from build123d import *

# Parameters (mm, degrees)
F1_DEPTH  = 1875
F2_W      = 2
F2_H      = 28
F3_DEPTH  = 650
F4_W      = 500
F4_H      = 400
F5_DEPTH  = 300
F6_W      = 496
F6_H      = 396
F7_DEPTH  = 300
F8_R      = 50
F9_R      = 50
F10_R     = 25
F11_DEPTH = 2
F12_R     = 12.5
F13_DEPTH = 2
F14_W     = 30
F14_H     = 30
F15_DEPTH = 920
F16_W     = 570
F16_H     = 30
F17_DEPTH = 1815


with BuildPart() as f1:
    # F0 (on Right) → F1 (new body)
    with BuildSketch(Plane.YZ):
        Polygon((0, 30), (0, 0), (700, 0), (700, 80), (680, 80), (680, 2), (30, 2), (30, 30), align=None)
    extrude(amount=F1_DEPTH)

    # F2 (on face) → F3 (join, through all)
    with BuildSketch(Plane(origin=(0, 30, 0), x_dir=(-1, 0, 0), z_dir=(0, 1, 0))):
        with Locations((-1874, 16)):
            Rectangle(F2_W, F2_H)
        with Locations((-1, 16)):
            Rectangle(F2_W, F2_H)
    extrude(amount=F3_DEPTH)

    # F4 (on face) → F5 (join)
    with BuildSketch(Plane(origin=(0, 0, 0), x_dir=(1, 0, 0), z_dir=(0, 0, -1))):
        with Locations((650, -300)):
            Rectangle(F4_W, F4_H)
        with Locations((1200, -300)):
            Rectangle(F4_W, F4_H)
    extrude(amount=F5_DEPTH)

    # F6 (on face) → F7 (cut)
    with BuildSketch(Plane.XY.offset(2)):
        with Locations((650, 300)):
            Rectangle(F6_W, F6_H)
        with Locations((1200, 300)):
            Rectangle(F6_W, F6_H)
    extrude(amount=-F7_DEPTH, mode=Mode.SUBTRACT)

    # F8
    f8_edges = [f1.edges().sort_by_distance(p)[0] for p in [
        (402, 102, -148),
        (402, 498, -148),
        (952, 498, -148),
        (1448, 498, -148),
        (898, 498, -148),
        (898, 102, -148),
        (1448, 102, -148),
        (1448, 300, -298),
        (1200, 498, -298),
        (952, 300, -298),
        (952, 102, -148),
        (1200, 102, -298),
        (650, 102, -298),
        (402, 300, -298),
        (650, 498, -298),
        (898, 300, -298),
    ]]
    fillet(f8_edges, radius=F8_R)

    # F9
    f9_edges = [f1.edges().sort_by_distance(p)[0] for p in [
        (400, 100, -150),
        (900, 100, -150),
        (950, 100, -150),
        (1450, 100, -150),
        (1450, 500, -150),
        (950, 500, -150),
        (900, 500, -150),
        (400, 500, -150),
        (400, 300, -300),
        (650, 500, -300),
        (900, 300, -300),
        (650, 100, -300),
        (950, 300, -300),
        (1200, 500, -300),
        (1450, 300, -300),
        (1200, 100, -300),
    ]]
    fillet(f9_edges, radius=F9_R)

    # F10 (on face) → F11 (cut, through all)
    with BuildSketch(Plane.XY.offset(-298)):
        with Locations((650, 373)):
            Circle(F10_R)
        with Locations((1200, 373)):
            Circle(F10_R)
    extrude(amount=-F11_DEPTH, mode=Mode.SUBTRACT)

    # F12 (on face) → F13 (cut, through all)
    with BuildSketch(Plane.XY.offset(2)):
        with Locations((560, 588)):
            Circle(F12_R)
        with Locations((740, 588)):
            Circle(F12_R)
        with Locations((1110, 588)):
            Circle(F12_R)
        with Locations((1290, 588)):
            Circle(F12_R)
    extrude(amount=-F13_DEPTH, mode=Mode.SUBTRACT)

    # F14 (on face) → F15 (join)
    with BuildSketch(Plane(origin=(0, 0, 0), x_dir=(1, 0, 0), z_dir=(0, 0, -1))):
        with Locations((45, -45)):
            Rectangle(F14_W, F14_H)
        with Locations((1830, -45)):
            Rectangle(F14_W, F14_H)
        with Locations((1830, -585)):
            Rectangle(F14_W, F14_H)
        with Locations((45, -585)):
            Rectangle(F14_W, F14_H)
    extrude(amount=F15_DEPTH)

    # F16 (on face) → F17 (join, through all)
    with BuildSketch(Plane.YZ.offset(1845)):
        with Locations((315, -785)):
            Rectangle(F16_W, F16_H)
    extrude(amount=-F17_DEPTH)


solid = f1.part
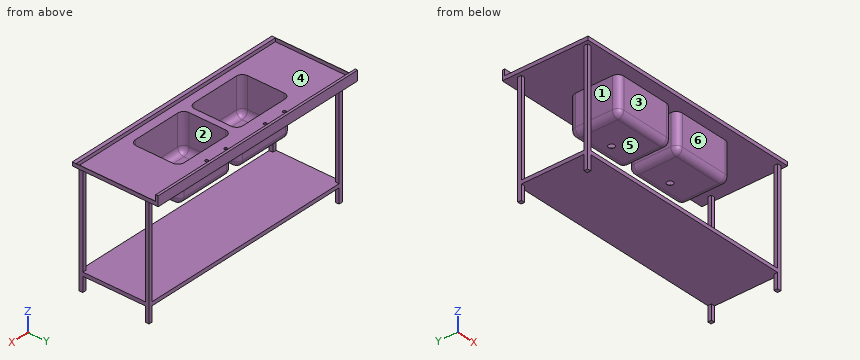
Can you work these out from the model? Positions are in its coordinate system, mm. Face numbers are marked on the shaded views. A direction names the side the tool comes from. Coordinates: 2 decimals unless noted, no trailing zeros. Write each loop counter-clockwise with the first axis right and the second up, starting at its lowest first coordinate (ties: lowest second). Pieces come first, ordered by that corner, then holes. Notation, with made-up numbers: (58.5, 53.5) - (80.5, 53.5) arc R21 cw to (80.5, 80.5) - close; hole circle Ø3 at (75.5, 68.25). An arc over 180 degrees is marked (long way). Return JSON: item names as keys, results as strings. Group by question number.
Item 1: Which directions (+Z, -Z, +X, -X, +Y, -Y) give clear straight access to the entire face, cutting with the end or side of a thin tool? Please do the marked faces 4, 5 and 6.
Item 2: We'd pull the mould along X, two halves only. Please class the marked faces 1, 2 and 3: pulls with the +X half, pulls with the -X half, needs draft (parallel to the pull), parting line crosses it, or undercut.
Item 3: If we section it at A-A (x = 1200): Write out the boundary of the cut face in (y, z).
Item 4: If we section it at D-D (z = -24): Count the separate pieces of the cut face and the enclosed holes in it, then the cut area to 3 significant figures.
Item 5: If we section it at C-C (x = 792.5): Write out the boundary of the cut face in (y, z), then the cut area to 3 significant figures.
Item 6: If we section it at B-B (z = -422): Write out the boundary of the cut face in (x, y).
Item 7: Please list where these lines run through material, in increasing order: probe 1 along X at (y, z) = (588, 1); probe 2 along Y at (x, z) = (1290, 0.5); probe 3 along Z at (x, y) = (1334, 62.5).
Item 8: I'm going to push flat-ended pins straight in: pin 1 Ø3 at (x, y) = (770.5, 628) entering from +Z; pin 2 Ø15 at (y, z) = (49, -271.5) entering from +X; pin 3 Ø8 at (x, z) = (1168.5, -149) entering from +Y. Where does each tip first touch, or does it pass through?
Return value:
{
 "1": {"face 4": "+Z", "face 5": "+X, -X, +Y, -Y", "face 6": "+X, -X, -Y"},
 "2": {"face 1": "pulls with the -X half", "face 2": "undercut", "face 3": "needs draft"},
 "3": {"outline": "(0, 0) - (100, 0) - (100, -250) arc R50 ccw to (150, -300) - (348, -300) - (348, -298) - (152, -298) arc R50 cw to (102, -248) - (102, 2) - (30, 2) - (30, 30) - (0, 30) - close; (30, -800) - (600, -800) - (600, -770) - (30, -770) - close; (398, -300) - (450, -300) arc R50 ccw to (500, -250) - (500, 0) - (700, 0) - (700, 80) - (680, 80) - (680, 2) - (498, 2) - (498, -248) arc R50 cw to (448, -298) - (398, -298) - close"},
 "4": {"separate pieces": "6", "enclosed holes": "2", "area": "10,800 mm^2"},
 "5": {"outline": "(0, 0) - (100, 0) - (100, -250) arc R50 ccw to (150, -300) - (450, -300) arc R50 ccw to (500, -250) - (500, 0) - (700, 0) - (700, 80) - (680, 80) - (680, 2) - (498, 2) - (498, -248) arc R50 cw to (448, -298) - (152, -298) arc R50 cw to (102, -248) - (102, 2) - (30, 2) - (30, 30) - (0, 30) - close; (30, -800) - (600, -800) - (600, -770) - (30, -770) - close", "area": "22,100 mm^2"},
 "6": {"outline": "(30, 30) - (60, 30) - (60, 60) - (30, 60) - close; (30, 570) - (60, 570) - (60, 600) - (30, 600) - close; (1815, 30) - (1845, 30) - (1845, 60) - (1815, 60) - close; (1815, 570) - (1845, 570) - (1845, 600) - (1815, 600) - close"},
 "7": {"probe 1": "x = 0 to 547.5, 572.5 to 727.5, 752.5 to 1097.5, 1122.5 to 1277.5, 1302.5 to 1875", "probe 2": "y = 0 to 102, 498 to 575.5, 600.5 to 700", "probe 3": "z = -800 to -770, 0 to 2"},
 "8": {"pin 1": "stops at z = 2", "pin 2": "stops at x = 1845", "pin 3": "stops at y = 500"}
}
